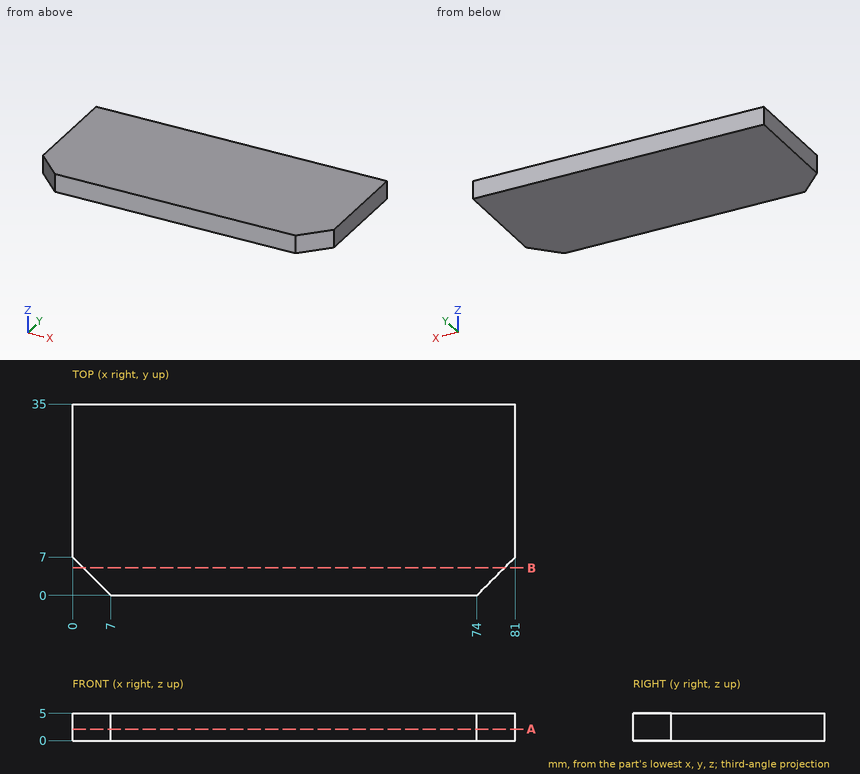
Here's the drawing with two shaded views (mm, measured from the low corner). I have some questions. Round coordinates to 2 decimals unless told otherwise and drop trailing zeros. Loops run counter-clockwise (first coordinate to the right, second up) from the corner with the lowest first, then second, coordinate; pieces in that order, holes last.
Item 1: Suppose I cut it at A-A, the plane z = 2.1. Write out the boundary of the cut face in (x, y), then the cut area to 3 significant figures.
Item 2: Suppose I cut it at B-B, the plane y = 5. Write out the boundary of the cut face in (x, z), then the cut area to 3 significant figures.
Item 3: Please list where these lines run through material, in increasing order: L1, parallel to X at y = 4, z = 2.75; L2, parallel to X at y = 2.5, z = 2.8; L3, parallel to Y at x = 78, z = 2.65.
Reported:
1. outline: (0, 7) - (7, 0) - (74, 0) - (81, 7) - (81, 35) - (0, 35) - close
1. area: 2,790 mm2
2. outline: (2, 0) - (79, 0) - (79, 5) - (2, 5) - close
2. area: 385 mm2
3. L1: x = 3 to 78
3. L2: x = 4.5 to 76.5
3. L3: y = 4 to 35
